Part model, mm, in its own coordinate system. A direction names the side the tool comes from. Round coordinates to 2 decimals unless told otherwise and drop trailing zeros. Write each loop counter-clockwise with the first axis right and the second up, starting at its lowest first coordinate (ties: lowest second). Pieces come first, ordered by that corner, then holes.
Solid Edge part; units mm, degrees
sketch "Sketch1" plane through (0, 0, 0) normal (0, 0, 1) x (1, 0, 0)
  circle A0 centre (0, 0) radius 12.5
extrude "ExtrudedProtrusion_1" add sketch "Sketch1" against normal blind 9
sketch "Sketch2" plane through (0, 0, 0) normal (0, 0, 1) x (1, 0, 0)
  circle A0 centre (0, 0) radius 8
extrude "ExtrudedProtrusion_2" add sketch "Sketch2" along normal blind 96
sketch "Sketch3" plane through (0, 0, 0) normal (0, -1, 0) x (1, 0, 0)
  line L0 (15, 89) -> (15, 91)
  line L1 (15, 91) -> (-15, 90)
  line L2 (-15, 90) -> (-15, 89)
  line L3 (15, 89) -> (-15, 89)
  line L4 (0, 89) -> (15, 89)
revolve "RevolvedCutout1" cut sketch "Sketch3" angle 360 about axis through (0, 0, 89) along (1, 0, 0)
Q1. Which spindle directions (+Z, -Z, +X, -X, +Y, -Y) get a long thin tool onto all of the face, cutting with end or side? Do faces 4 (the flat face through (-0.2, -8.2, 0)), 5 (the flat face through (0, 0, 96)). Say none if no direction does.
Values follow:
face 4: +Z
face 5: +Z, +X, -X, +Y, -Y
Q2. Mould opens along Z. For faces 1 (the flat face through (0, 0, -9)), 2 (the cylindrical face through (11.923, 3.755, -4.437)), 3 (the conical face through (0.112, -1.016, 87.892)) say: +Z half, -Z half, draft (parallel to the pull), parting line (faces both ways), or undercut.
Values follow:
face 1: -Z half
face 2: draft
face 3: undercut
Q3. Wall check: L1, parallel to Z at x = 8.5, y = 7; L2, parallel to Z at x = 4.5, y = -0.75; L3, parallel to X at y = -5, z = 67 (3 decimals). Give the ranges that are in metal, low to high.
Values follow:
L1: z = -9 to 0
L2: z = -9 to 87.53, 90.47 to 96
L3: x = -6.245 to 6.245
Q4. Drop flat-ended pins along their axis: pin 1 (5 mm diameter, centred on y = 8, z = 28.5, fed in from +X); pin 2 (8 mm diameter, centred on x = -8.5, z = 7, fed in from -Y); pin 3 (12 mm diameter, centred on x = 1.5, z = 26, fed in from +Y). Give the stop position or say it passes through.
Values follow:
pin 1: stops at x = 5.81
pin 2: stops at y = -6.61
pin 3: stops at y = 8
Q5. Cut at A-A on x = 0. Write the cut outline in (y, z), plus the area to 3 significant figures.
Values follow:
outline: (-12.5, -9) - (12.5, -9) - (12.5, 0) - (8, 0) - (8, 96) - (-8, 96) - (-8, 0) - (-12.5, 0) - close; hole circle Ø3 at (0, 89)
area: 1,750 mm2
Q6. Cut at C-C on z = 89. Write the cut outline in (x, y), plus the area to 3 significant figures.
Values follow:
outline: (-7.9, -1.24) arc R8 ccw to (7.8, -1.76) - close; (-7.9, 1.24) - (7.8, 1.76) arc R8 ccw to start
area: 153 mm2
Q7. Cut at D-D on y = -5.5. Write the cut outline in (x, z).
Values follow:
outline: (-11.22, -9) - (11.22, -9) - (11.22, 0) - (5.81, 0) - (5.81, 96) - (-5.81, 96) - (-5.81, 0) - (-11.22, 0) - close
Q8. Cut at B-B on y = 0. Write the cut outline in (x, z).
Values follow:
outline: (-12.5, -9) - (12.5, -9) - (12.5, 0) - (8, 0) - (8, 87.23) - (-8, 87.77) - (-8, 0) - (-12.5, 0) - close; (-8, 90.23) - (8, 90.77) - (8, 96) - (-8, 96) - close
